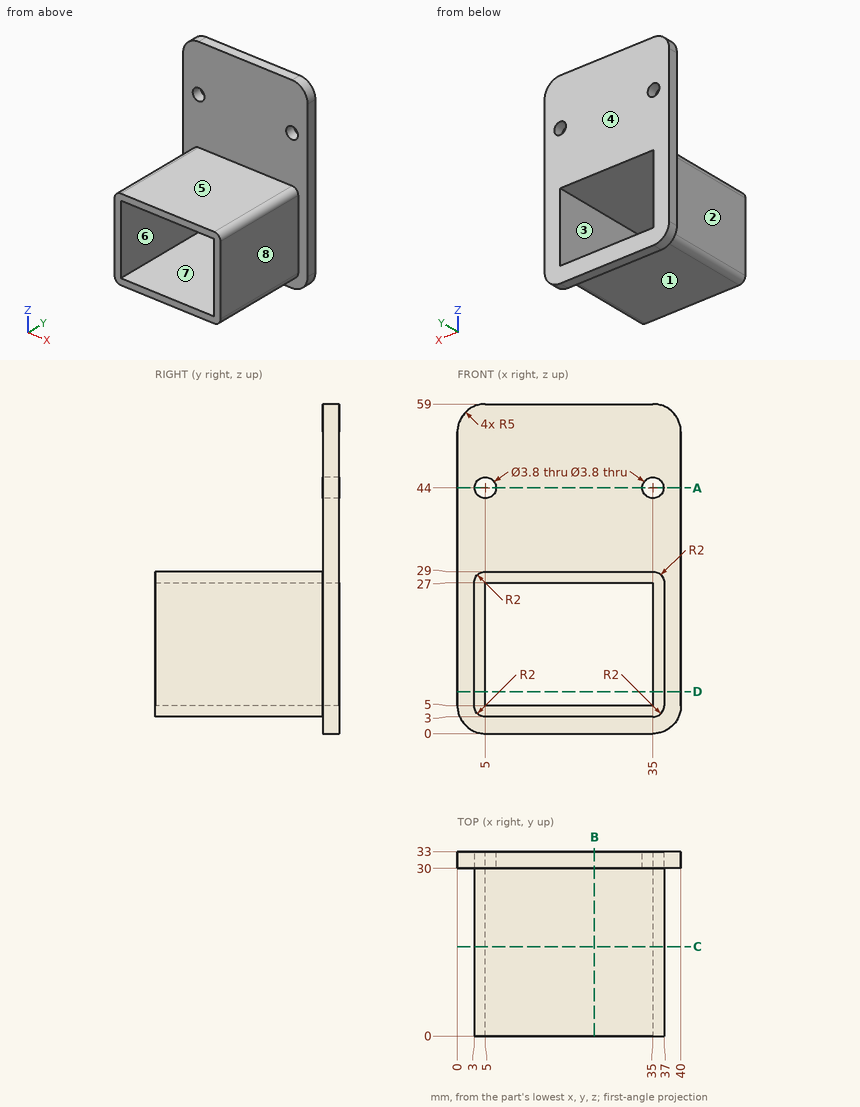
Here's the drawing with two shaded views (mm, measured from the low corner). I have some questions. A direction names the side the tool comes from. Coordinates: 2 decimals unless noted, no trailing zeros. Loops run counter-clockwise (first coordinate to the right, second up) from the corner with the lowest first, then second, coordinate; pieces in that order, holes last. Notation, with made-up numbers: (-1, 84) -> (42, 84) arc R23 cw to (42, 114) -> close; hole circle Ø2 at (50, -33). An arc over 180 degrees is marked (long way). Answer in a Markdown table with one row per item.
(1) Imagine slicing it at D-D (z = 7.5). List the corners of the cut face in (x, y) for me, plus the area to 3 significant figures.
Results found:
| item | result |
|---|---|
| outline | (0, 30) -> (3, 30) -> (3, 0) -> (5, 0) -> (5, 33) -> (0, 33) -> close; (35, 0) -> (37, 0) -> (37, 30) -> (40, 30) -> (40, 33) -> (35, 33) -> close |
| area | 150 mm^2 |
(2) Thinking about a two-plate mould opening in Z: for the marked faces 5, 6, 7 and 8, which applies, released by +Z, released by -Z, zero draft, split by the parting line, or undercut?
Results found:
| item | result |
|---|---|
| face 5 | released by +Z |
| face 6 | undercut |
| face 7 | undercut |
| face 8 | zero draft |
(3) For the marked faces 1, 2, 3 and 4, which set-ups out of +Z, -Z, +X, -X, +Y, -Y let a thin tool reach every point of the face, with its end or its side?
Results found:
| item | result |
|---|---|
| face 1 | -Z, +X, -X, -Y |
| face 2 | +Z, -Z, -X, -Y |
| face 3 | +Y, -Y |
| face 4 | +Z, -Z, +X, -X, +Y |
(4) If I drill on probe 1 along X at (y, z) = (21.5, 13.5); probe 2 along Z at (x, y) = (12.5, 16.5); probe 3 along Y at (x, z) = (38, 49.5), over which ranges is the centre line in solid material (lowest first)?
Results found:
| item | result |
|---|---|
| probe 1 | x = 3 to 5, 35 to 37 |
| probe 2 | z = 3 to 5, 27 to 29 |
| probe 3 | y = 30 to 33 |
(5) Imagine slicing it at C-C (y = 16). List the corners of the cut face in (x, z) for me.
Results found:
| item | result |
|---|---|
| outline | (3, 5) arc R2 ccw to (5, 3) -> (35, 3) arc R2 ccw to (37, 5) -> (37, 27) arc R2 ccw to (35, 29) -> (5, 29) arc R2 ccw to (3, 27) -> close; hole (5, 5) -> (35, 5) -> (35, 27) -> (5, 27) -> close |
(6) Will these pins go through, and if not, where does the flat tip stop? pin 1 Ø8 at (y, z) = (8, 10.5) entering from -X; pin 2 Ø10 at (x, y) = (6, 7) entering from -Z; pin 3 Ø5 at (x, z) = (5, 44) entering from -Y.
Results found:
| item | result |
|---|---|
| pin 1 | stops at x = 3 |
| pin 2 | stops at z = 3 |
| pin 3 | stops at y = 30 |
(7) Imagine slicing it at A-A (z = 44). List the corners of the cut face in (x, y) for me, plus the area to 3 significant figures.
Results found:
| item | result |
|---|---|
| outline | (0, 30) -> (3.1, 30) -> (3.1, 33) -> (0, 33) -> close; (6.9, 30) -> (33.1, 30) -> (33.1, 33) -> (6.9, 33) -> close; (36.9, 30) -> (40, 30) -> (40, 33) -> (36.9, 33) -> close |
| area | 97.2 mm^2 |
(8) Imagine slicing it at B-B (x = 24.5). List the corners of the cut face in (y, z) for me, plus the area to 3 significant figures.
Results found:
| item | result |
|---|---|
| outline | (0, 3) -> (30, 3) -> (30, 0) -> (33, 0) -> (33, 5) -> (0, 5) -> close; (0, 27) -> (33, 27) -> (33, 59) -> (30, 59) -> (30, 29) -> (0, 29) -> close |
| area | 231 mm^2 |
